from build123d import *

# Parameters (mm, degrees)
SKETCH1_R                = 3.75
BOSS_EXTRUDE1_DEPTH      = 14
BOSS_EXTRUDE1_DEPTH_BACK = 9
BOSS_EXTRUDE2_DEPTH      = 3


with BuildPart() as part:
    # Sketch1 → Boss-Extrude1 (new body, two sides)
    with BuildSketch(Plane.ZY.offset(-65.969208633)) as boss_extrude1_sk:
        with Locations((-5.344766421, 7.785620452)):
            Circle(SKETCH1_R)
    extrude(amount=BOSS_EXTRUDE1_DEPTH)
    extrude(boss_extrude1_sk.sketch, amount=-BOSS_EXTRUDE1_DEPTH_BACK)

    # Sketch2 → Boss-Extrude2 (add)
    with BuildSketch(Plane.ZY.offset(-51.969208633)):
        Polygon((-9.094766421, 11.42591126), (-7.738890169, 12.781787511), (-2.950642672, 12.781787511), (-1.594766421, 11.42591126), (-0.237121401, 10.06826624), (-0.237121401, 5.502974665), (-1.594766421, 4.145329645), (-2.950642672, 2.789453394), (-7.738890169, 2.789453394), (-9.094766421, 4.145329645), (-10.45241144, 5.502974665), (-10.45241144, 10.06826624), align=None)
    extrude(amount=-BOSS_EXTRUDE2_DEPTH)


solid = part.part
Geometry check sheet. Reference: the model listing, model coordinates, mm. A direction names the side the tool comes from. Round coordinates to 2 decimals unless told otherwise and drop trailing zeros. Order: outer loops, then holes, each group sorted by start corner. A loop starts at its lowest first (then second) coordinate and runs counter-clockwise, first axis right, second up. Notation, with made-up numbers: M 0.25,11.5 L 27.25,11.5 A8 ccw 27.25,23.5 Z; hole C -25.75,31 d2. An arc over 180 degrees is marked long. Write each question's results on one line, items separated by ' | '. Start each with the question number.
1. Cross-section at A-A on y = 4.75. Record the boundary of the cut face in (x, z).
2. Cross-section at B-B on z = -4. Record the boundary of the cut face in (x, y), plus the area to 3 significant figures.
3. Material ranges on L1, parallel to X at y = 4.25, z = -3; L2, parallel to Y at x = 69.75, z = -6.25; L3, parallel to Z at x = 68.75, y = 8, recorded low to high. Write a range as from..to.
4. Cross-section at C-C on x = 69. Record the boundary of the cut face in (y, z), plus the area to 3 significant figures.
5. Go/stop test with flat-tipped pins: P1, Ø2, axis at x = 59, y = 8, coming from the +Z side; P2, Ø3, axis at x = 70.5, z = -5, coming from the +Y side; P3, Ø5, axis at x = 61, z = -9, coming from the +Y side. Record where each tip stops, or that it passes through.
6. Set-up check for faces 1 (the face through (64.83, 10.95, -3.33)), 2 (the face through (53, 2.789, -5)): record each of +Z, -Z, +X, -X, +Y, -Y from which the full face is reachable in a straight line by a thin tool's end or side.
Resolved:
1) outline: M 51.97,-9.7 L 54.97,-9.7 L 54.97,-7.55 L 74.97,-7.55 L 74.97,-3.14 L 54.97,-3.14 L 54.97,-0.99 L 51.97,-0.99 Z
2) outline: M 51.97,2.79 L 54.97,2.79 L 54.97,4.29 L 74.97,4.29 L 74.97,11.29 L 54.97,11.29 L 54.97,12.78 L 51.97,12.78 Z | area: 170 mm2
3) L1: 51.97..54.97 | L2: 4.15..11.42 | L3: -9.09..-1.6
4) outline: C 7.79,-5.34 d7.5 | area: 44.2 mm2
5) P1: z = -1.59 | P2: y = 11.54 | P3: y = 11.35
6) face 1: +X | face 2: +Z, -Z, +X, -X, -Y
